Design review of the part built by this model. Coordinates are the model's own, in mm. Face numbers are marked on the shaded views. A direction names the side the tool comes from. Round coordinates to 2 decimals unless told otherwise and drop trailing zeros. Loops run counter-clockwise (first coordinate to the right, second up) from the corner with the lowest first, then second, coordinate; pieces in that order, holes last. Notation, with made-up numbers: M -5,61 L 11,61 A30 cw 11,96 Z; hole C 79,71.25 d8. An arc over 180 degrees is marked long. Answer as CSV lines item,"result". Start each with the question number.
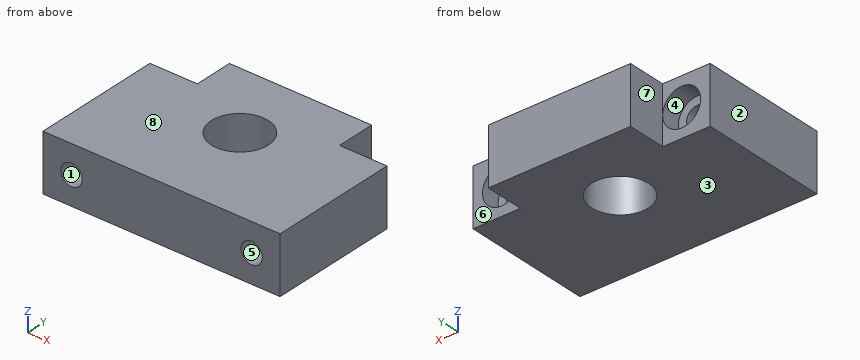
from build123d import *

# Parameters (mm, degrees)
SKETCH_1_W                   = 50
SKETCH_1_H                   = 27.3
EXTRUDE_1_DEPTH              = 12
SKETCH_2_W                   = 30
SKETCH_2_H                   = 30
EXTRUDE_2_DEPTH              = 12
SKETCH_3_R                   = 6
CUT_EXTRUDE_1_DEPTH          = 63.483997951
HOLE_WIZARD_M4_3_D           = 4.5
HOLE_WIZARD_M4_3_CBORE_D     = 8
HOLE_WIZARD_M4_3_CBORE_DEPTH = 4


with BuildPart() as part:
    # 스케치1 → 보스-돌출1 (new body)
    with BuildSketch(Plane.XY):
        with Locations((25, 13.65)):
            Rectangle(SKETCH_1_W, SKETCH_1_H)
    extrude(amount=EXTRUDE_1_DEPTH)

    # 스케치2 → 보스-돌출2 (add)
    with BuildSketch(Plane.XY.offset(12)):
        with Locations((25, 20.5)):
            Rectangle(SKETCH_2_W, SKETCH_2_H)
    extrude(amount=-EXTRUDE_2_DEPTH)

    # 스케치3 → 컷-돌출1 (cut, through all)
    with BuildSketch(Plane(origin=(0, 0, 0), x_dir=(-1, 0, 0), z_dir=(0, 0, -1))):
        with Locations((-25, 20)):
            Circle(SKETCH_3_R)
    extrude(amount=-CUT_EXTRUDE_1_DEPTH, mode=Mode.SUBTRACT)

    # M4 소켓 머리 캡 나사용 카운터보어3 (through all)
    with Locations(Plane(origin=(0, 27.3, 0), x_dir=(1, 0, 0), z_dir=(0, 1, 0))):
        with Locations((44, -6), (6, -6)):
            CounterBoreHole(HOLE_WIZARD_M4_3_D / 2, HOLE_WIZARD_M4_3_CBORE_D / 2, HOLE_WIZARD_M4_3_CBORE_DEPTH)


solid = part.part
Item 1: Consider section C-C, the plane z = 5. Write out the cut boundary in (x, y).
Item 2: Insertion check: pin 1 Ø2 at (y, z) = (11, 9) entering from -X; pin 2 Ø6 at (x, z) = (6, 6) entering from +Y. Each pin has a flat end and moves straight along its axis. Give the tip position at first contact, or say it passes through.
Item 3: Consider section B-B, the plane x = 25. Write out the cut boundary in (y, z), then the cut area to 3 significant figures.
Item 4: To check wall thickness, follow line 1 (Z direction, x = 44, y = 25); line 2 (Z direction, x = 44, y = 22); line 3 (X direction, y = 15, z = 6.5). State the ranges of each line that lie inside material, in increasing order.
Item 5: Consider section D-D, the plane z = 11. Write out the cut boundary in (x, y), then the cut area to 3 significant figures.
Item 6: The part is to be moulded in two halves that separate along Z. For the marked faces 1, 2 and 3, say which applies: +Z half, -Z half, draft (parallel to the pull), parting line (faces both ways), or undercut.
Item 7: Consider section A-A, the plane y = 20. Write out the cut boundary in (x, z).
Item 8: Tool access review of the marked faces 4, 5, 6, 7 and 8: name each direction out of +Z, -Z, +X, -X, +Y, -Y from which nothing blocks a thin tool from reaching the whole face with its end or side.
Found:
1,outline,"M 0,0 L 3.98,0 L 3.98,23.3 L 2.13,23.3 L 2.13,27.3 L 0,27.3 Z; M 8.02,0 L 41.98,0 L 41.98,23.3 L 40.13,23.3 L 40.13,27.3 L 40,27.3 L 40,35.5 L 10,35.5 L 10,27.3 L 9.87,27.3 L 9.87,23.3 L 8.02,23.3 Z; M 46.02,0 L 50,0 L 50,27.3 L 47.87,27.3 L 47.87,23.3 L 46.02,23.3 Z; hole C 25,20 d12"
2,pin 1,"stops at x = 0"
2,pin 2,"stops at y = 23.3"
3,outline,"M 0,0 L 14,0 L 14,12 L 0,12 Z; M 26,0 L 35.5,0 L 35.5,12 L 26,12 Z"
3,area,"282 mm^2"
4,line 1,"z = 0 to 2, 10 to 12"
4,line 2,"z = 0 to 3.75, 8.25 to 12"
4,line 3,"x = 0 to 3.81, 8.19 to 21.68, 28.32 to 41.81, 46.19 to 50"
5,outline,"M 0,0 L 50,0 L 50,27.3 L 40,27.3 L 40,35.5 L 10,35.5 L 10,27.3 L 0,27.3 Z; hole C 25,20 d12"
5,area,"1,500 mm^2"
6,face 1,"undercut"
6,face 2,"draft"
6,face 3,"-Z half"
7,outline,"M 0,0 L 19,0 L 19,12 L 0,12 Z; M 31,0 L 50,0 L 50,12 L 31,12 Z; hole C 6,6 d4.5; hole C 44,6 d4.5"
8,face 4,"+Y"
8,face 5,"+Y, -Y"
8,face 6,"+Z, -Z, +X, +Y"
8,face 7,"+Z, -Z, -X, +Y"
8,face 8,"+Z, +X, -X, +Y, -Y"
